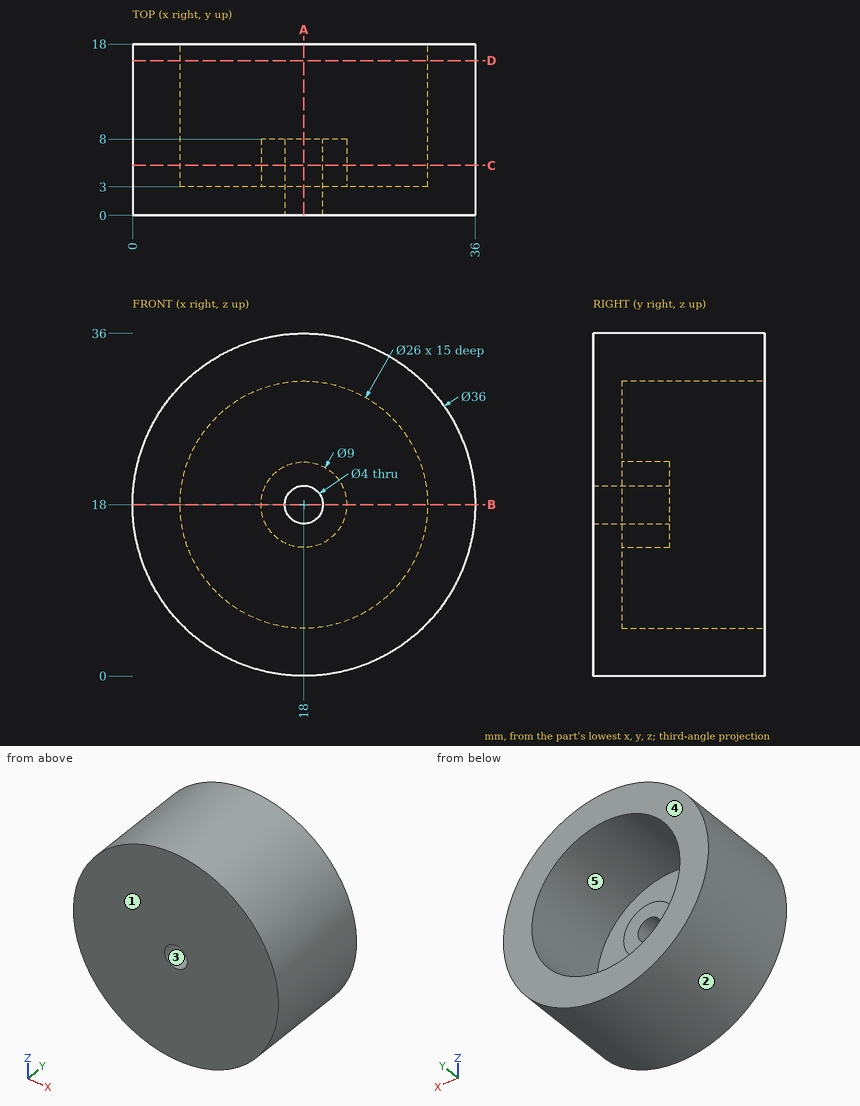
Check sheet for the drawn part. Datum: minimum x, y, z corner. Units: mm. A direction names the side the tool comes from. Coordinates: 2 decimals unless noted, no trailing zeros. Loops run counter-clockwise (first coordinate to the right, second up) from the corner with the lowest first, then second, coordinate; pieces in that order, holes last. Notation, with made-up numbers: (31, 21) -> (56, 21) arc R29 cw to (56, 52) -> close; hole circle Ø5 at (30.25, -35). An arc over 180 degrees is marked (long way). Write each question's results on one line, items separated by ' | '.
Item 1: Gauge pin test, flat ends, axial feed: pin 1 (6 mm diameter, centred on y = 4.5, z = 6.5, fed in from +X); pin 2 (3 mm diameter, centred on y = 14, z = 30.5, fed in from +X); pin 3 (3 mm diameter, centred on x = 20, y = 3.5, fed in from -Z). Record the tip position at first contact, or that the pin passes through.
Found:
pin 1: stops at x = 33.87 | pin 2: stops at x = 32.25 | pin 3: stops at z = 0.01
Item 2: Section check A-A, the plane x = 18. Enter the section's corners in (y, z).
Found:
outline: (0, 0) -> (18, 0) -> (18, 5) -> (3, 5) -> (3, 13.5) -> (8, 13.5) -> (8, 16) -> (0, 16) -> close; (0, 20) -> (8, 20) -> (8, 22.5) -> (3, 22.5) -> (3, 31) -> (18, 31) -> (18, 36) -> (0, 36) -> close
Item 3: Section check B-B, the plane z = 18. Enter the section's corners in (x, y).
Found:
outline: (0, 0) -> (16, 0) -> (16, 8) -> (13.5, 8) -> (13.5, 3) -> (5, 3) -> (5, 18) -> (0, 18) -> close; (20, 0) -> (36, 0) -> (36, 18) -> (31, 18) -> (31, 3) -> (22.5, 3) -> (22.5, 8) -> (20, 8) -> close
Item 4: Tool access check on the marked faces 4 and 5. Record the directions out of +Z, -Z, +X, -X, +Y, -Y that give a thin tool (end or side, any length) a straight path to the whole face; none if there is none.
Found:
face 4: +Z, -Z, +X, -X, +Y | face 5: +Y
Item 5: Section check D-D, the plane y = 16.25. Enter the section's corners in (x, z).
Found:
outline: circle Ø36 at (18, 18); hole circle Ø26 at (18, 18)
Item 6: Section check C-C, the plane y = 5.25. Enter the section's corners in (x, z).
Found:
outline: circle Ø36 at (18, 18); circle Ø9 at (18, 18); hole circle Ø26 at (18, 18); hole circle Ø4 at (18, 18)
Item 7: Material ranges on L1, parallel to X at y = 7, z = 21; L2, parallel to Z at x = 14, y = 7; L3, parallel to X at y = 10.75, z = 18, recorded low to high.
Found:
L1: x = 0.25 to 5.35, 14.65 to 21.35, 30.65 to 35.75 | L2: z = 0.45 to 5.63, 15.94 to 20.06, 30.37 to 35.55 | L3: x = 0 to 5, 31 to 36
Item 8: Mould release check, pull along Z, two halves, no side actions. Record for the marked faces 1, 2 and 3: +Z half, -Z half, draft (parallel to the pull), parting line (faces both ways), or undercut.
Found:
face 1: draft | face 2: parting line | face 3: undercut
